Source: CAD feature listing. Evaluate the final solid. Frame: model axes, mm. Give positions to 0.01 mm unless a question says otherwise; leave off trailing zeros. Loops run counter-clockwise (first coordinate to the right, second up) from the corner with the lowest first, then second, coordinate; pieces in that order, holes last.
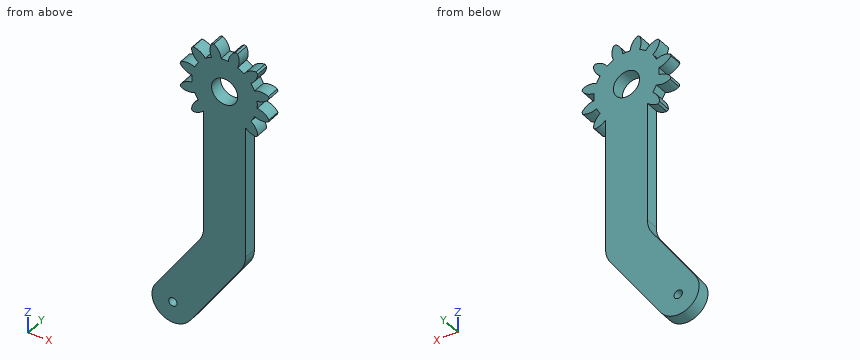
from build123d import *

# Parameters (mm, degrees)
BOSS_EXTRUDE1_DEPTH = 5
FILLET1_RADIUS      = 8
FILLET1_LENGTH      = 5
FILLET2_R           = 10
SKETCH2_R           = 1.6
CUT_EXTRUDE2_DEPTH  = 103.399978443
BOSS_EXTRUDE3_DEPTH = 5
SKETCH6_R           = 5
CUT_EXTRUDE3_DEPTH  = 103.399978443


with BuildPart() as part:
    # Sketch1 → Boss-Extrude1 (new body)
    with BuildSketch(Plane(origin=(0, 0, 0), x_dir=(1, 0, 0), z_dir=(0, 1, 0))):
        with BuildLine():
            Line((8, 9.604686356), (8, 64.67016599))
            Line((8, 64.67016599), (-17.836624745, 101.568690121))
            Line((-17.836624745, 101.568690121), (-30.943057454, 92.391467139))
            Line((-30.943057454, 92.391467139), (-8, 59.625385368))
            Line((-8, 59.625385368), (-8, 9.604686356))
            ThreePointArc((-8, 9.604686356), (0, -12.5), (8, 9.604686356))
        make_face()
    extrude(amount=BOSS_EXTRUDE1_DEPTH)

    # Fillet1: full round fillet: the end face becomes a half cylinder, R = half its width
    fillet1_face = Plane((-24.3898411, 2.5, -96.98007863), x_dir=(0, 1, 0), z_dir=(-0.573576436351, 0, -0.819152044289))  # on the end face: x along it, z out of the body
    fillet1_slab = fillet1_face.offset(-FILLET1_RADIUS / 2) * Box(FILLET1_LENGTH, 2 * FILLET1_RADIUS, FILLET1_RADIUS, mode=Mode.PRIVATE)  # the body's end, R deep
    fillet1_round = Plane((-19.801229609, 2.5, -90.426862276), x_dir=(-0.573576436351, 0, -0.819152044289), z_dir=(0, 1, 0)) * Cylinder(FILLET1_RADIUS, FILLET1_LENGTH, mode=Mode.PRIVATE)  # its axis R under the face
    add(fillet1_slab - fillet1_round, mode=Mode.SUBTRACT)

    # Fillet2
    fillet2_edges = [part.edges().sort_by_distance(p)[0] for p in [
        (-8, 2.5, -59.625385368),
        (8, 2.5, -64.67016599),
    ]]
    fillet(fillet2_edges, radius=FILLET2_R)

    # Sketch2 → Cut-Extrude2 (cut, through all)
    with BuildSketch(Plane(origin=(0, 5, 0), x_dir=(1, 0, 0), z_dir=(0, 1, 0))):
        with Locations(Location((-19.801229609, 90.426862276, 0), (0, 0, 270))):
            Circle(SKETCH2_R)
    extrude(amount=-CUT_EXTRUDE2_DEPTH, mode=Mode.SUBTRACT)

    # Sketch5 → Boss-Extrude3 (add)
    with BuildSketch(Plane(origin=(0, 5, 0), x_dir=(1, 0, 0), z_dir=(0, 1, 0))):
        with BuildLine():
            ThreePointArc((-12.051706508, -12.688828561), (-9.162245044, -11.749370601), (-7.103491322, -9.514845613))
            ThreePointArc((-7.103491322, -9.514845613), (-5.937, -10.283185645), (-4.688352353, -10.909226747))
            ThreePointArc((-4.688352353, -10.909226747), (-5.594130897, -13.809422264), (-4.962994624, -16.781498275))
            ThreePointArc((-4.962994624, -16.781498275), (-4.529333289, -16.90370196), (-4.092669715, -17.014701132))
            ThreePointArc((-4.092669715, -17.014701132), (-2.060051663, -14.756375941), (-1.394381134, -11.791843675))
            ThreePointArc((-1.394381134, -11.791843675), (0, -11.874), (1.394381134, -11.791843675))
            ThreePointArc((1.394381134, -11.791843675), (2.060051663, -14.756375941), (4.092669715, -17.014701132))
            ThreePointArc((4.092669715, -17.014701132), (4.529333289, -16.90370196), (4.962994624, -16.781498275))
            ThreePointArc((4.962994624, -16.781498275), (5.594130897, -13.809422264), (4.688352353, -10.909226747))
            ThreePointArc((4.688352353, -10.909226747), (5.937, -10.283185645), (7.103491322, -9.514845613))
            ThreePointArc((7.103491322, -9.514845613), (9.162245044, -11.749370601), (12.051706508, -12.688828561))
            ThreePointArc((12.051706508, -12.688828561), (12.374368671, -12.374368671), (12.688828561, -12.051706508))
            ThreePointArc((12.688828561, -12.051706508), (11.749370601, -9.162245044), (9.514845613, -7.103491322))
            ThreePointArc((9.514845613, -7.103491322), (10.283185645, -5.937), (10.909226747, -4.688352353))
            ThreePointArc((10.909226747, -4.688352353), (13.809422264, -5.594130897), (16.781498275, -4.962994624))
            ThreePointArc((16.781498275, -4.962994624), (16.90370196, -4.529333289), (17.014701132, -4.092669715))
            ThreePointArc((17.014701132, -4.092669715), (14.756375941, -2.060051663), (11.791843675, -1.394381134))
            ThreePointArc((11.791843675, -1.394381134), (11.874, 0), (11.791843675, 1.394381134))
            ThreePointArc((11.791843675, 1.394381134), (14.756375941, 2.060051663), (17.014701132, 4.092669715))
            ThreePointArc((17.014701132, 4.092669715), (16.90370196, 4.529333289), (16.781498275, 4.962994624))
            ThreePointArc((16.781498275, 4.962994624), (13.809422264, 5.594130897), (10.909226747, 4.688352353))
            ThreePointArc((10.909226747, 4.688352353), (10.283185645, 5.937), (9.514845613, 7.103491322))
            ThreePointArc((9.514845613, 7.103491322), (11.749370601, 9.162245044), (12.688828561, 12.051706508))
            ThreePointArc((12.688828561, 12.051706508), (12.374368671, 12.374368671), (12.051706508, 12.688828561))
            ThreePointArc((12.051706508, 12.688828561), (9.162245044, 11.749370601), (7.103491322, 9.514845613))
            ThreePointArc((7.103491322, 9.514845613), (5.937, 10.283185645), (4.688352353, 10.909226747))
            ThreePointArc((4.688352353, 10.909226747), (5.594130897, 13.809422264), (4.962994624, 16.781498275))
            ThreePointArc((4.962994624, 16.781498275), (4.529333289, 16.90370196), (4.092669715, 17.014701132))
            ThreePointArc((4.092669715, 17.014701132), (2.060051663, 14.756375941), (1.394381134, 11.791843675))
            ThreePointArc((1.394381134, 11.791843675), (0, 11.874), (-1.394381134, 11.791843675))
            ThreePointArc((-1.394381134, 11.791843675), (-2.060051663, 14.756375941), (-4.092669715, 17.014701132))
            ThreePointArc((-4.092669715, 17.014701132), (-4.529333289, 16.90370196), (-4.962994624, 16.781498275))
            ThreePointArc((-4.962994624, 16.781498275), (-5.594130897, 13.809422264), (-4.688352353, 10.909226747))
            ThreePointArc((-4.688352353, 10.909226747), (-5.937, 10.283185645), (-7.103491322, 9.514845613))
            ThreePointArc((-7.103491322, 9.514845613), (-9.162245044, 11.749370601), (-12.051706508, 12.688828561))
            ThreePointArc((-12.051706508, 12.688828561), (-12.374368671, 12.374368671), (-12.688828561, 12.051706508))
            ThreePointArc((-12.688828561, 12.051706508), (-11.749370601, 9.162245044), (-9.514845613, 7.103491322))
            ThreePointArc((-9.514845613, 7.103491322), (-10.283185645, 5.937), (-10.909226747, 4.688352353))
            ThreePointArc((-10.909226747, 4.688352353), (-13.809422264, 5.594130897), (-16.781498275, 4.962994624))
            ThreePointArc((-16.781498275, 4.962994624), (-16.90370196, 4.529333289), (-17.014701132, 4.092669715))
            ThreePointArc((-17.014701132, 4.092669715), (-14.756375941, 2.060051663), (-11.791843675, 1.394381134))
            ThreePointArc((-11.791843675, 1.394381134), (-11.874, 0), (-11.791843675, -1.394381134))
            ThreePointArc((-11.791843675, -1.394381134), (-14.756375941, -2.060051663), (-17.014701132, -4.092669715))
            ThreePointArc((-17.014701132, -4.092669715), (-16.90370196, -4.529333289), (-16.781498275, -4.962994624))
            ThreePointArc((-16.781498275, -4.962994624), (-13.809422264, -5.594130897), (-10.909226747, -4.688352353))
            ThreePointArc((-10.909226747, -4.688352353), (-10.283185645, -5.937), (-9.514845613, -7.103491322))
            ThreePointArc((-9.514845613, -7.103491322), (-11.749370601, -9.162245044), (-12.688828561, -12.051706508))
            ThreePointArc((-12.688828561, -12.051706508), (-12.374368671, -12.374368671), (-12.051706508, -12.688828561))
        make_face()
    extrude(amount=-BOSS_EXTRUDE3_DEPTH)

    # Sketch6 → Cut-Extrude3 (cut, through all)
    with BuildSketch(Plane(origin=(0, 5, 0), x_dir=(1, 0, 0), z_dir=(0, 1, 0))):
        with Locations(Location((0, 0, 0), (0, 0, 270))):
            Circle(SKETCH6_R)
    extrude(amount=-CUT_EXTRUDE3_DEPTH, mode=Mode.SUBTRACT)


solid = part.part
1) Cut plane C-C (x = 0). Return loops of the section in (y, z).
Checks:
outline: (0, -76.1) - (5, -76.1) - (5, -5) - (0, -5) - close; (0, 5) - (5, 5) - (5, 12.5) - (0, 12.5) - close
2) Ray query, probe 1 along Z at (x, y) = (-10.5, 1.25); probe 2 along X at (y, z) = (1, -54); probe 3 along Z at (x, y) = (-14.5, 4.35). Return the intervals inside material, ascending.
Checks:
probe 1: z = -91.09 to -63.2, -12.39 to -7.76, -6.78 to 6.78, 7.76 to 12.39
probe 2: x = -8 to 8
probe 3: z = -96.42 to -68.91, -5.59 to -1.94, 1.94 to 5.59
3) Contact query for flat-ended pins moving along their axis: P1, Ø2, axis at y = 1, z = -59, coming from the +X side; P2, Ø1, axis at y = 2.5, z = -86, coming from the -X side; P3, Ø16, axis at x = 0, z = 0, coming from the -Y side; P4, Ø1.5, axis at x = -12, y = 3.5, coming from the +Z side. Output: stop coordinate, or through.
Checks:
P1: stops at x = 8
P2: stops at x = -26.77
P3: stops at y = 0
P4: stops at z = 12.69
4) Cut plane D-D (z = -30). Return loops of the section in (x, y).
Checks:
outline: (-8, 0) - (8, 0) - (8, 5) - (-8, 5) - close
5) Cut plane B-B (x = -14.5). Return loops of the section in (y, z).
Checks:
outline: (0, -96.42) - (5, -96.42) - (5, -68.91) - (0, -68.91) - close; (0, -5.59) - (5, -5.59) - (5, -1.94) - (0, -1.94) - close; (0, 1.94) - (5, 1.94) - (5, 5.59) - (0, 5.59) - close
6) Cut plane A-A (z = 0). Return loops of the section in (x, y).
Checks:
outline: (-12.5, 0) - (-5, 0) - (-5, 5) - (-12.5, 5) - close; (5, 0) - (12.5, 0) - (12.5, 5) - (5, 5) - close
